from build123d import *

# Parameters (mm, degrees)
PAD_DEPTH       = 6
SKETCH001_W     = 5.4
SKETCH001_H     = 2.5
SKETCH001_W_2   = 2.7
POCKET_DEPTH    = 250.237688
SKETCH002_R     = 1.7
POCKET001_DEPTH = 250.237688


with BuildPart() as part:
    # Sketch → Pad (new body)
    with BuildSketch(Plane.YZ):
        Polygon((-50, 30), (-35, 30), (-35, 0), (35, 0), (35, 30), (50, 30), (50, 20), (56, 20), (56, -2.3), (50, -2.3), (50, -12.3), (40, -12.3), (40, -18.3), (18, -18.3), (18, -12.3), (-18, -12.3), (-18, -18.3), (-40, -18.3), (-40, -12.3), (-50, -12.3), (-50, -2.3), (-56, -2.3), (-56, 20), (-50, 20), align=None)
    extrude(amount=PAD_DEPTH)

    # Sketch001 (on Face25 of Pad) → Pocket (cut, through all)
    with BuildSketch(Plane(origin=(0, 0, 0), x_dir=(0, 1, 0), z_dir=(-1, 0, 0))):
        with Locations((45, 8.05)):
            Rectangle(SKETCH001_W, SKETCH001_H)
        with Locations((1.35, 8.05)):
            Rectangle(SKETCH001_W_2, SKETCH001_H)
    pocket = extrude(amount=-POCKET_DEPTH, mode=Mode.SUBTRACT)

    # Mirrored: Pocket across Sketch001 V_Axis
    add(pocket.mirror(Plane(origin=(0, 0, 0), x_dir=(-1, 0, 0), z_dir=(0, 1, 0))), mode=Mode.SUBTRACT)

    # Sketch002 (on Face4 of Mirrored) → Pocket001 (cut, through all)
    with BuildSketch(Plane(origin=(0, 0, 0), x_dir=(0, 1, 0), z_dir=(-1, 0, 0))):
        with Locations((53, -15)):
            Circle(SKETCH002_R)
        with Locations((53, -2.7)):
            Circle(SKETCH002_R)
    pocket001 = extrude(amount=-POCKET001_DEPTH, mode=Mode.SUBTRACT)

    # Mirrored001: Pocket001 across Sketch002 V_Axis
    add(pocket001.mirror(Plane(origin=(0, 0, 0), x_dir=(-1, 0, 0), z_dir=(0, 1, 0))), mode=Mode.SUBTRACT)


solid = part.part
Could you check a few things on this model? Use its own coordinates, in mm. A direction names the side the tool comes from. Coordinates: 2 decimals unless noted, no trailing zeros. Write each loop counter-clockwise with the first axis right and the second up, starting at its lowest first coordinate (ties: lowest second). Pieces come first, ordered by that corner, then holes. Notation, with made-up numbers: (-21, 8) - (-17, 8) arc R14 ccw to (-17, 32) - close; hole circle Ø8 at (26, -8.75). An arc over 180 degrees is marked (long way). Write item = value, one per line.
1) Suppose I cut it at B-B on z = 2.7. Please give me the cut outline in (x, y).
Result set:
outline = (0, -56) - (6, -56) - (6, -54.7) - (0, -54.7) - close; (0, -51.3) - (6, -51.3) - (6, -35) - (0, -35) - close; (0, 35) - (6, 35) - (6, 51.3) - (0, 51.3) - close; (0, 54.7) - (6, 54.7) - (6, 56) - (0, 56) - close
2) For faces 5 (the flat face through (3, -50, -7)), 6 (the flat face through (3, 0, 0)), 7 (the flat face through (3, 50, -7)), which set-ups out of +Z, -Z, +X, -X, +Y, -Y let a thin tool reach every point of the face, with its end or its side?
Result set:
face_5 = -Z, +X, -X, -Y
face_6 = +Z, +X, -X
face_7 = -Z, +X, -X, +Y
3) Suppose I cut it at C-C on z = -14.5. Please give me the cut outline in (x, y), plus the area to 3 significant figures.
Result set:
outline = (0, -40) - (6, -40) - (6, -18) - (0, -18) - close; (0, 18) - (6, 18) - (6, 40) - (0, 40) - close
area = 264 mm2
4) Will these pins go through, and if not, where does the flat tip stop? pin 1 Ø3 at (x, y) = (2.5, 1.5) entering from +Z; pin 2 Ø4 at (y, z) = (-53, 15) entering from -X; pin 3 Ø1.8 at (x, y) = (1.5, -54.5) entering from +Z; pin 4 Ø0.8 at (x, z) = (2.5, -8.5) entering from -Y.
Result set:
pin_1 = 0
pin_2 = 0
pin_3 = 20
pin_4 = -50
5) We'd pull the mould along Z, two halves only. Please class faces 1 (the flat face through (3, 18, -15)), 2 (the flat face through (3, 53, 20)), 3 (the cylindrical face through (2.96, -51.3, 14.93)), 4 (the flat face through (3, 53, -2.3)): +Z half, -Z half, draft (parallel to the pull), parting line (faces both ways), or undercut.
Result set:
face_1 = draft
face_2 = +Z half
face_3 = undercut
face_4 = -Z half
6) Please list where these lines run through material, in increasing order: line 1 (Y direction, x = 2.55, z = 2.7); line 2 (Z direction, x = 3.85, y = -53); line 3 (Y direction, x = 3.4, z = 23.5). Write a range as [from, to].
Result set:
line_1 = [-56, -54.7], [-51.3, -35], [35, 51.3], [54.7, 56]
line_2 = [-2.3, 1], [4.4, 13.3], [16.7, 20]
line_3 = [-50, -35], [35, 50]
7) Suppose I cut it at A-A on y = 53. Please give me the cut outline in (x, z), plus the area to 3 significant figures.
Result set:
outline = (0, -2.3) - (6, -2.3) - (6, 1) - (0, 1) - close; (0, 4.4) - (6, 4.4) - (6, 13.3) - (0, 13.3) - close; (0, 16.7) - (6, 16.7) - (6, 20) - (0, 20) - close
area = 93.0 mm2
8) Suppose I cut it at D-D on x = 4.75. State how many separate pieces and enclosed holes the cut face has, plus the area to 3 significant figures.
Result set:
separate_pieces = 1
enclosed_holes = 7
area = 2,580 mm2
